```python
from build123d import *

# Parameters (mm, degrees)
CROQUIS1_W              = 74
CROQUIS1_H              = 80
SALIENTE_EXTRUIR1_DEPTH = 10
CROQUIS2_W              = 65.8
CROQUIS2_H              = 4
CORTAR_EXTRUIR1_DEPTH   = 60
CROQUIS3_W              = 45
CROQUIS3_H              = 60
CORTAR_EXTRUIR3_DEPTH   = 39
CROQUIS6_W              = 30.164087926
CROQUIS6_H              = 10
SALIENTE_EXTRUIR3_DEPTH = 15
REDONDEO1_R             = 10
REDONDEO2_R             = 10
CROQUIS7_R              = 1.8
CORTAR_EXTRUIR5_DEPTH   = 32
REDONDEO3_R             = 10
REDONDEO4_R             = 10
REDONDEO5_R             = 10
REDONDEO6_R             = 10


with BuildPart() as part:
    # Croquis1 → Saliente-Extruir1 (new body)
    with BuildSketch(Plane.XY):
        Rectangle(CROQUIS1_W, CROQUIS1_H)
    extrude(amount=SALIENTE_EXTRUIR1_DEPTH)

    # Croquis2 → Cortar-Extruir1 (cut)
    with BuildSketch(Plane.XZ.offset(40)):
        with Locations((0, 5)):
            Rectangle(CROQUIS2_W, CROQUIS2_H)
    extrude(amount=-CORTAR_EXTRUIR1_DEPTH, mode=Mode.SUBTRACT)

    # Croquis3 → Cortar-Extruir3 (cut)
    with BuildSketch(Plane.XY.offset(10)):
        with Locations((0, -10)):
            Rectangle(CROQUIS3_W, CROQUIS3_H)
    extrude(amount=-CORTAR_EXTRUIR3_DEPTH, mode=Mode.SUBTRACT)

    # Croquis6 → Saliente-Extruir3 (add)
    with BuildSketch(Plane(origin=(0, 40, 0), x_dir=(1, 0, 0), z_dir=(0, 1, 0))):
        with Locations((0, -5)):
            Rectangle(CROQUIS6_W, CROQUIS6_H)
    extrude(amount=SALIENTE_EXTRUIR3_DEPTH)

    # Redondeo1
    redondeo1_edges = [part.edges().sort_by_distance(p)[0] for p in [
        (-37, 40, 5),
    ]]
    fillet(redondeo1_edges, radius=REDONDEO1_R)

    # Redondeo2
    redondeo2_edges = [part.edges().sort_by_distance(p)[0] for p in [
        (37, 40, 5),
    ]]
    fillet(redondeo2_edges, radius=REDONDEO2_R)

    # Croquis7 → Cortar-Extruir5 (cut)
    with BuildSketch(Plane.ZY.offset(15.082043963)):
        with Locations((5, 50)):
            Circle(CROQUIS7_R)
    extrude(amount=-CORTAR_EXTRUIR5_DEPTH, mode=Mode.SUBTRACT)

    # Redondeo3
    redondeo3_edges = [part.edges().sort_by_distance(p)[0] for p in [
        (-22.5, 20, 8.5),
    ]]
    fillet(redondeo3_edges, radius=REDONDEO3_R)

    # Redondeo4
    redondeo4_edges = [part.edges().sort_by_distance(p)[0] for p in [
        (-22.5, 20, 1.5),
    ]]
    fillet(redondeo4_edges, radius=REDONDEO4_R)

    # Redondeo5
    redondeo5_edges = [part.edges().sort_by_distance(p)[0] for p in [
        (22.5, 20, 8.5),
    ]]
    fillet(redondeo5_edges, radius=REDONDEO5_R)

    # Redondeo6
    redondeo6_edges = [part.edges().sort_by_distance(p)[0] for p in [
        (22.5, 20, 1.5),
    ]]
    fillet(redondeo6_edges, radius=REDONDEO6_R)


solid = part.part
```
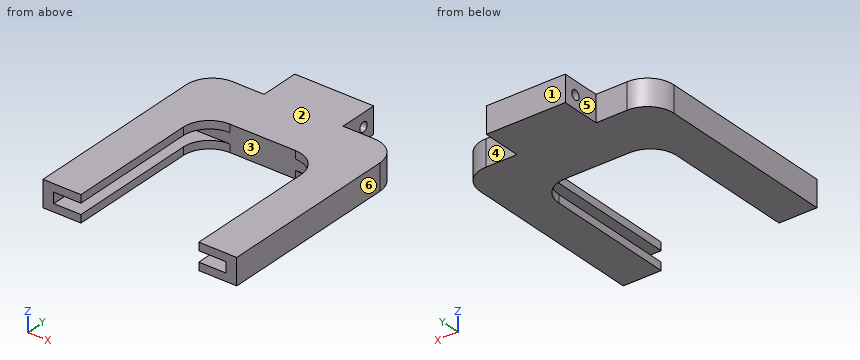
Design review of the part built by this model. Coordinates are the model's own, in mm. Face numbers are marked on the shaded views. A direction names the side the tool comes from. Give positions to 0.01 mm unless a question says otherwise; leave off trailing zeros. Write each loop counter-clockwise with the first axis right and the second up, starting at its lowest first coordinate (ties: lowest second). Pieces come first, ordered by that corner, then holes.
(1) Tool access review of the marked faces 4, 5 and 6: name each direction out of +Z, -Z, +X, -X, +Y, -Y from which nothing blocks a thin tool from reaching the whole face with its end or side.
Checked values:
face 4: +Z, -Z, +X, +Y
face 5: +Z, -Z, -X, +Y
face 6: +Z, -Z, +X, +Y, -Y
(2) Add section A-A (y = -8). Give the boundary of the cut face in (x, z), and give its area (3 significant figures).
Checked values:
outline: (-37, 0) - (-22.5, 0) - (-22.5, 3) - (-32.9, 3) - (-32.9, 7) - (-22.5, 7) - (-22.5, 10) - (-37, 10) - close; (22.5, 0) - (37, 0) - (37, 10) - (22.5, 10) - (22.5, 7) - (32.9, 7) - (32.9, 3) - (22.5, 3) - close
area: 207 mm2
(3) Add section D-D (y = 50). Give the boundary of the cut face in (x, z), and give its area (3 significant figures).
Checked values:
outline: (-15.08, 0) - (15.08, 0) - (15.08, 3.2) - (-15.08, 3.2) - close; (-15.08, 6.8) - (15.08, 6.8) - (15.08, 10) - (-15.08, 10) - close
area: 193 mm2
(4) Add section C-C (x = -24.5). Give the boundary of the cut face in (y, z), and give its area (3 significant figures).
Checked values:
outline: (-40, 0) - (40, 0) - (40, 10) - (-40, 10) - (-40, 7) - (20, 7) - (20, 3) - (-40, 3) - close
area: 560 mm2
(5) Mouldability with a two-part tool opening along Z and no side actions: class the marked faces 1, 2 and 3 as +Z half, -Z half, draft (parallel to the pull), parting line (faces both ways), or undercut.
Checked values:
face 1: draft
face 2: +Z half
face 3: undercut
(6) Clearance check with flat-ended pins moving along their axes: pin 1 Ø3 at (y, z) = (46.5, 4) entering from -X; pin 2 Ø3 at (y, z) = (50, 5) entering from -X; pin 3 Ø4 at (x, z) = (-26, 9) entering from +Y; pin 4 Ø3 at (x, z) = (-25, 5) entering from -Y. State where each tip first meets the part, or that it passes through.
Checked values:
pin 1: stops at x = -15.08
pin 2: passes through
pin 3: stops at y = 40
pin 4: stops at y = 20
(7) Add section B-B (z = 5). Give the boundary of the cut face in (x, y).
Checked values:
outline: (-37, -40) - (-32.9, -40) - (-32.9, 20) - (32.9, 20) - (32.9, -40) - (37, -40) - (37, 30) arc R10 ccw to (27, 40) - (15.08, 40) - (15.08, 48.2) - (-15.08, 48.2) - (-15.08, 40) - (-27, 40) arc R10 ccw to (-37, 30) - close; (-15.08, 51.8) - (15.08, 51.8) - (15.08, 55) - (-15.08, 55) - close
(8) Wall thickness on line 1 along X through (y, z) = (-19.5, 0.5); line 2 along Y through (x, z) = (2, 5); line 3 along Y through (x, z) = (-7.5, 1.75): over which ranges is each line inside the solid? List them lowest first.
Checked values:
line 1: x = -37 to -22.5, 22.5 to 37
line 2: y = 20 to 48.2, 51.8 to 55
line 3: y = 20 to 55
